from build123d import *

# Parameters (mm, degrees)
SKETCH_1_W                         = 27
SKETCH_1_H                         = 1
SM_BASE_FLANGE_1_DEPTH             = 85
SM_EDGE_FLANGE_1_STRIP_W           = 5.4732
SM_EDGE_FLANGE_1_STRIP_H           = 1
SM_EDGE_FLANGE_1_STRIP_CUT_DEPTH   = 85
SM_EDGE_FLANGE_1_STRIP_2_W         = 5.4732
SM_EDGE_FLANGE_1_STRIP_2_H         = 1
SM_EDGE_FLANGE_1_STRIP_CUT_2_DEPTH = 85
SM_EDGE_FLANGE_1_DEPTH             = 85
SM_EDGE_FLANGE_1_BEND_DEPTH        = 85
SM_EDGE_FLANGE_2_STRIP_W           = 5.4732
SM_EDGE_FLANGE_2_STRIP_H           = 1
SM_EDGE_FLANGE_2_STRIP_CUT_DEPTH   = 85
SM_EDGE_FLANGE_2_STRIP_2_W         = 5.4732
SM_EDGE_FLANGE_2_STRIP_2_H         = 1
SM_EDGE_FLANGE_2_STRIP_CUT_2_DEPTH = 85
SM_EDGE_FLANGE_2_DEPTH             = 85
SM_EDGE_FLANGE_2_BEND_DEPTH        = 85
CUT_EXTRUDE_2_DEPTH                = 88.025858226
CUT_EXTRUDE_1_REACH                = 89.026
OTHER_3_DEPTH                      = 1


# Read off the part's stored shape, not the designer's step: Образец заполнения3
# Sheet-metal steps are written as plain solids
with BuildPart() as part:
    # Sketch 1 → Базовая кромка1 (new body)
    with BuildSketch(Plane.XY):
        with Locations((0, 0.5)):
            Rectangle(SKETCH_1_W, SKETCH_1_H)
    extrude(amount=SM_BASE_FLANGE_1_DEPTH)

    # Ребро-кромка1 strip (across the edge) → Ребро-кромка1 strip cut (cut)
    with BuildSketch(Plane(origin=(-13.5, 1, 0), x_dir=(1, 0, 0), z_dir=(0, 0, 1))):
        with Locations((-1, -0.5)):
            Rectangle(SM_EDGE_FLANGE_1_STRIP_W, SM_EDGE_FLANGE_1_STRIP_H)
    extrude(amount=SM_EDGE_FLANGE_1_STRIP_CUT_DEPTH, mode=Mode.SUBTRACT)

    # Ребро-кромка1 strip 2 (across the edge) → Ребро-кромка1 strip cut 2 (cut)
    with BuildSketch(Plane(origin=(13.5, 1, 85), x_dir=(-1, 0, 0), z_dir=(0, 0, -1))):
        with Locations((-1, -0.5)):
            Rectangle(SM_EDGE_FLANGE_1_STRIP_2_W, SM_EDGE_FLANGE_1_STRIP_2_H)
    extrude(amount=SM_EDGE_FLANGE_1_STRIP_CUT_2_DEPTH, mode=Mode.SUBTRACT)

    # Ребро-кромка1 section (across the edge) → Ребро-кромка1 (add)
    with BuildSketch(Plane(origin=(-13.5, 1, 0), x_dir=(1, 0, 0), z_dir=(0, 0, 1))):
        with BuildLine():
            Line((0, 0.7366), (0, 6.5))
            Line((0, 6.5), (1, 6.5))
            Line((1, 6.5), (1, 0.7366))
            ThreePointArc((1, 0.7366), (1.215745145, 0.215745145), (1.7366, 0))
            Line((1.7366, 0), (1.7366, -1))
            ThreePointArc((1.7366, -1), (0.508638364, -0.491361636), (0, 0.7366))
        make_face()
    extrude(amount=SM_EDGE_FLANGE_1_DEPTH)

    # Ребро-кромка1 section 2 (across the edge) → Ребро-кромка1 bend (add)
    with BuildSketch(Plane(origin=(13.5, 1, 85), x_dir=(-1, 0, 0), z_dir=(0, 0, -1))):
        with BuildLine():
            Line((0, 0.7366), (0, 6.5))
            Line((0, 6.5), (1, 6.5))
            Line((1, 6.5), (1, 0.7366))
            ThreePointArc((1, 0.7366), (1.215745145, 0.215745145), (1.7366, 0))
            Line((1.7366, 0), (1.7366, -1))
            ThreePointArc((1.7366, -1), (0.508638364, -0.491361636), (0, 0.7366))
        make_face()
    extrude(amount=SM_EDGE_FLANGE_1_BEND_DEPTH)

    # Ребро-кромка2 strip (across the edge) → Ребро-кромка2 strip cut (cut)
    with BuildSketch(Plane(origin=(-13.5, 7.5, 85), x_dir=(0, -1, 0), z_dir=(0, 0, -1))):
        with Locations((-1, -0.5)):
            Rectangle(SM_EDGE_FLANGE_2_STRIP_W, SM_EDGE_FLANGE_2_STRIP_H)
    extrude(amount=SM_EDGE_FLANGE_2_STRIP_CUT_DEPTH, mode=Mode.SUBTRACT)

    # Ребро-кромка2 strip 2 (across the edge) → Ребро-кромка2 strip cut 2 (cut)
    with BuildSketch(Plane(origin=(13.5, 7.5, 0), x_dir=(0, -1, 0), z_dir=(0, 0, 1))):
        with Locations((-1, -0.5)):
            Rectangle(SM_EDGE_FLANGE_2_STRIP_2_W, SM_EDGE_FLANGE_2_STRIP_2_H)
    extrude(amount=SM_EDGE_FLANGE_2_STRIP_CUT_2_DEPTH, mode=Mode.SUBTRACT)

    # Ребро-кромка2 section (across the edge) → Ребро-кромка2 (add)
    with BuildSketch(Plane(origin=(-13.5, 7.5, 85), x_dir=(0, -1, 0), z_dir=(0, 0, -1))):
        with BuildLine():
            Line((0, 0.7366), (0, 4))
            Line((0, 4), (1, 4))
            Line((1, 4), (1, 0.7366))
            ThreePointArc((1, 0.7366), (1.215745145, 0.215745145), (1.7366, 0))
            Line((1.7366, 0), (1.7366, -1))
            ThreePointArc((1.7366, -1), (0.508638364, -0.491361636), (0, 0.7366))
        make_face()
    extrude(amount=SM_EDGE_FLANGE_2_DEPTH)

    # Ребро-кромка2 section 2 (across the edge) → Ребро-кромка2 bend (add)
    with BuildSketch(Plane(origin=(13.5, 7.5, 0), x_dir=(0, -1, 0), z_dir=(0, 0, 1))):
        with BuildLine():
            Line((0, 0.7366), (0, 4))
            Line((0, 4), (1, 4))
            Line((1, 4), (1, 0.7366))
            ThreePointArc((1, 0.7366), (1.215745145, 0.215745145), (1.7366, 0))
            Line((1.7366, 0), (1.7366, -1))
            ThreePointArc((1.7366, -1), (0.508638364, -0.491361636), (0, 0.7366))
        make_face()
    extrude(amount=SM_EDGE_FLANGE_2_BEND_DEPTH)

    # Эскиз19 → Вырез-Вытянуть2 (cut, through all)
    with BuildSketch(Plane(origin=(0, 1, 0), x_dir=(1, 0, 0), z_dir=(0, 1, 0))):
        with BuildLine():
            Line((-1.370314889, 0), (1.370314889, 0))
            ThreePointArc((1.370314889, 0), (0, -0.54321), (-1.370314889, 0))
        make_face()
        with BuildLine():
            Line((-1.370314889, -85), (1.370314889, -85))
            ThreePointArc((1.370314889, -85), (0, -84.45679), (-1.370314889, -85))
        make_face()
    extrude(amount=-CUT_EXTRUDE_2_DEPTH, mode=Mode.SUBTRACT)

    # Эскиз18 → Вырез-Вытянуть1 (cut, up to next)
    with BuildSketch(Plane(origin=(0, 1, 0), x_dir=(1, 0, 0), z_dir=(0, 1, 0)), mode=Mode.PRIVATE) as cut_extrude_1_sk1:
        with BuildLine():
            Line((-2, -18), (-2, -10))
            ThreePointArc((-2, -10), (0, -8), (2, -10))
            Line((2, -10), (2, -18))
            ThreePointArc((2, -18), (0, -20), (-2, -18))
        make_face()
    cut_extrude_1_tool1 = extrude(cut_extrude_1_sk1.sketch, amount=-CUT_EXTRUDE_1_REACH, mode=Mode.PRIVATE) & part.part
    add(cut_extrude_1_tool1.solids().sort_by_distance((0, 1, 14))[0], mode=Mode.SUBTRACT)

    # Образец заполнения3 outline → Образец заполнения3 (cut)
    with BuildSketch(Plane(origin=(0, 0, 0), x_dir=(1, 0, 0), z_dir=(0, 1, 0))):
        with BuildLine():
            ThreePointArc((2, -30), (0, -28), (-2, -30))
            Line((-2, -30), (-2, -38))
            ThreePointArc((-2, -38), (0, -40), (2, -38))
            Line((2, -38), (2, -30))
        make_face()
        with BuildLine():
            ThreePointArc((2, -70), (0, -68), (-2, -70))
            Line((-2, -70), (-2, -78))
            ThreePointArc((-2, -78), (0, -80), (2, -78))
            Line((2, -78), (2, -70))
        make_face()
        with BuildLine():
            ThreePointArc((2, -50), (0, -48), (-2, -50))
            Line((-2, -50), (-2, -58))
            ThreePointArc((-2, -58), (0, -60), (2, -58))
            Line((2, -58), (2, -50))
        make_face()
    extrude(amount=OTHER_3_DEPTH, mode=Mode.SUBTRACT)


solid = part.part
Geometry check sheet. Reference: the model listing, model coordinates, mm. A direction names the side the tool comes from. Round coordinates to 2 decimals unless told otherwise and drop trailing zeros. Order: outer loops, then holes, each group sorted by start corner. A loop starts at its lowest first (then second) coordinate and runs counter-clockwise, first axis right, second up. Notation, with made-up numbers: (-24.75, 70.25) - (6.25, 70.25) arc R26 cw to (6.25, 100.25) - close; hole circle Ø6 at (18.5, 17.5). An arc over 180 degrees is marked (long way). One line per question, with ' | ' between items. Start each with the question number.
(1) Sectioned sample at A-A on x = 0. Record the cut outline in (y, z).
(2) Release check for a two-part mould opening along X. For faces 5 (the flat face through (-13.5, 4, 42)), 6 (the cylindrical face through (0, 0.5, 28)), 7 (the flat face through (-16, 6.5, 43)), 8 (the flat face through (13.5, 4, 43)) record: released by +X, released by -X, zero draft, split by the parting line, or undercut.
(3) Depth check by flat-ended pin: pin 1 Ø2 at (y, z) = (4.5, 31) entering from +X; pin 2 Ø0.8 at (y, z) = (0.5, 74) entering from -X; pin 3 Ø0.8 at (y, z) = (0.5, 34.5) entering from +X. Enter the tip coordinate at first touch or a pass-through.
(4) Sectioned sample at D-D on z = 64. Record the cut outline in (x, y), and give its area (3 significant figures).
(5) Access from +Z, -Z, +X, -X, +Y, -Y to the whole of each face (thin tool, end or side, straight path). Record for faces 1 (the flat face through (16, 6.5, 42)), 2 (the cylindrical face through (13, 6.98, 41.9)), 3 (the cylindrical face through (0, 0.5, 40)), 4 (the flat face through (-10, 0.7, 0)).
(6) Sectioned sample at C-C on y = 5. Record the cut outline in (x, z).
(7) Thickness scan on L1, parallel to X at y = 2.25, z = 27; L2, parallel to Y at x = 2, z = 60; L3, parallel to Y at x = 15, z = 6.5. Record the ranges inside material, lowest first. Write a range as [from, to].
(8) Sectioned sample at B-B on z = 12. Record the cut outline in (x, y), and give its area (3 significant figures).
Conclusion:
1) outline: (0, 0.54) - (1, 0.54) - (1, 8) - (0, 8) - close; (0, 20) - (1, 20) - (1, 28) - (0, 28) - close; (0, 40) - (1, 40) - (1, 48) - (0, 48) - close; (0, 60) - (1, 60) - (1, 68) - (0, 68) - close; (0, 80) - (1, 80) - (1, 84.46) - (0, 84.46) - close
2) face 5: released by -X | face 6: undercut | face 7: zero draft | face 8: released by +X
3) pin 1: stops at x = 13.5 | pin 2: stops at x = -13.29 | pin 3: stops at x = 13.29
4) outline: (-17.5, 6.5) - (-14.24, 6.5) arc R0.74 cw to (-13.5, 5.76) - (-13.5, 1.74) arc R1.74 ccw to (-11.76, 0) - (11.76, 0) arc R1.74 ccw to (13.5, 1.74) - (13.5, 5.76) arc R0.74 cw to (14.24, 6.5) - (17.5, 6.5) - (17.5, 7.5) - (14.24, 7.5) arc R1.74 ccw to (12.5, 5.76) - (12.5, 1.74) arc R0.74 cw to (11.76, 1) - (-11.76, 1) arc R0.74 cw to (-12.5, 1.74) - (-12.5, 5.76) arc R1.74 ccw to (-14.24, 7.5) - (-17.5, 7.5) - close | area: 45.9 mm2
5) face 1: +Z, -Z, +X, -Y | face 2: +Z, -Z, +Y | face 3: +Y, -Y | face 4: -Z, +X, -X, +Y, -Y
6) outline: (-13.5, 0) - (-12.5, 0) - (-12.5, 85) - (-13.5, 85) - close; (12.5, 0) - (13.5, 0) - (13.5, 85) - (12.5, 85) - close
7) L1: x = [-13.5, -12.5], [12.5, 13.5] | L2: y = [0, 1] | L3: y = [6.5, 7.5]
8) outline: (-17.5, 6.5) - (-14.24, 6.5) arc R0.74 cw to (-13.5, 5.76) - (-13.5, 1.74) arc R1.74 ccw to (-11.76, 0) - (-2, 0) - (-2, 1) - (-11.76, 1) arc R0.74 cw to (-12.5, 1.74) - (-12.5, 5.76) arc R1.74 ccw to (-14.24, 7.5) - (-17.5, 7.5) - close; (2, 0) - (11.76, 0) arc R1.74 ccw to (13.5, 1.74) - (13.5, 5.76) arc R0.74 cw to (14.24, 6.5) - (17.5, 6.5) - (17.5, 7.5) - (14.24, 7.5) arc R1.74 ccw to (12.5, 5.76) - (12.5, 1.74) arc R0.74 cw to (11.76, 1) - (2, 1) - close | area: 41.9 mm2
